```python
from build123d import *

# Parameters (mm, degrees)
EXTRUDE_1_DEPTH   = 2
HOLE_WIZARD_M81_D = 9
CHAMFER_1_SIZE    = 2.5


with BuildPart() as part:
    # Эскиз3 → Бобышка-Вытянуть1 (new body)
    with BuildSketch(Plane(origin=(0, 0, 0), x_dir=(1, 0, 0), z_dir=(0, 0, -1))):
        Polygon((0, 0), (100, 0), (100, 129.289321881), (64.644660941, 164.644660941), (0, 100), align=None)
    extrude(amount=EXTRUDE_1_DEPTH)

    # Отверстие с зазором M81 (through all)
    with Locations(Plane(origin=(0, 0, -2), x_dir=(1, 0, 0), z_dir=(0, 0, -1))):
        with Locations((22.5, 22.5), (77.5, 22.5), (31.819805153, 100), (66.412427894, 134.59262274), (35.496760416, 100.141421356), (66.412427894, 131.057088834), (25, 22.5), (75, 22.5)):
            Hole(HOLE_WIZARD_M81_D / 2)

    # Фаска1
    chamfer_1_edges = [part.edges().sort_by_distance(p)[0] for p in [
        (64.644660941, -164.644660941, -1),
        (100, 0, -1),
        (0, 0, -1),
    ]]
    chamfer(chamfer_1_edges, length=CHAMFER_1_SIZE)


solid = part.part
```
The listing builds one solid part. Answer for the finished solid, in the listing's coordinates (mm). Round coordinates to 2 decimals unless told otherwise and drop trailing zeros. Loops run counter-clockwise (first coordinate to the right, second up) from the corner with the lowest first, then second, coordinate; pieces in that order, holes last. Notation, with made-up numbers: (25, 8) - (83, 8) arc R13 cw to (83, 15) - close; hole circle Ø9 at (41, 81). An arc over 180 degrees is marked (long way). Return JSON: item names as keys, results as strings. Group by question number.
1. The part is cut by section D-D on x = 8. Determine the outline of the cut face in (y, z), then the cut area to 3 significant figures.
2. The mould has two halves that part along Y. Classify faces 1 (the cylindrical face through (82, -22.6, -1)), 2 (the flat face through (49, -64, -2)), 3 (the flat face through (83.44, -145.85, -0.99)): pulls with the +Y half, pulls with the -Y half, needs draft (parallel to the pull), parting line crosses it, or undercut.
3. The part is cut by section C-C on z = -1.35. Determine the outline of the cut face in (x, y), then the cut area to 3 significant figures.
4. The part is cut by section B-B on y = -131. Determine the outline of the cut face in (x, z).
5. Consider probe 1 along Y at (x, z) = (69, -1.75); probe 2 along Y at (x, z) = (91, -1.1); probe 3 along Y at (x, z) = (81, -0.7). Determine where each line is inside the solid, lowest interval first.
6. The part is cut by section A-A on y = -22.5. Determine the outline of the cut face in (x, z).
Resolved:
{
 "1": {"outline": "(-108, -2) - (0, -2) - (0, 0) - (-108, 0) - close", "area": "216 mm²"},
 "2": {"face 1": "undercut", "face 2": "needs draft", "face 3": "pulls with the -Y half"},
 "3": {"outline": "(0, -100) - (62.88, -162.88) - (66.41, -162.88) - (100, -129.29) - (100, -2.5) - (97.5, 0) - (2.5, 0) - (0, -2.5) - close; hole (23.75, -26.82) arc R4.5 ccw (long way) to (23.75, -18.18) arc R4.5 ccw (long way) to start; hole (33.5, -104.17) arc R4.5 ccw (long way) to (33.82, -95.97) arc R4.5 ccw (long way) to start; hole (62.27, -132.82) arc R4.5 ccw (long way) to (70.55, -132.82) arc R4.5 ccw (long way) to start; hole (76.25, -26.82) arc R4.5 ccw (long way) to (76.25, -18.18) arc R4.5 ccw (long way) to start", "area": "13,400 mm²"},
 "4": {"outline": "(31, -2) - (61.91, -2) - (61.91, 0) - (31, 0) - close; (70.91, -2) - (98.29, -2) - (98.29, 0) - (70.91, 0) - close"},
 "5": {"probe 1": "y = -160.29 to -138.27, -127.38 to 0", "probe 2": "y = -138.29 to 0", "probe 3": "y = -148.29 to -25.33, -19.67 to 0"},
 "6": {"outline": "(0, -2) - (18, -2) - (18, 0) - (0, 0) - close; (29.5, -2) - (70.5, -2) - (70.5, 0) - (29.5, 0) - close; (82, -2) - (100, -2) - (100, 0) - (82, 0) - close"}
}
